Part model, mm, in its own coordinate system. Give positions to 0.01 mm unless a question says otherwise; leave off trailing zeros. Write each loop counter-clockwise with the first axis right and the second up, starting at its lowest first coordinate (ties: lowest second). Pieces come first, ordered by that corner, then holes.
from build123d import *

# Parameters (mm, degrees)
SKETCH1_W           = 25.4
SKETCH1_H           = 25.4
SKETCH1_W_2         = 22.225
SKETCH1_H_2         = 22.225
BOSS_EXTRUDE1_DEPTH = 228.6
SKETCH3_R           = 2.54
CUT_EXTRUDE2_DEPTH  = 232.40501291
SKETCH4_R           = 2.54
CUT_EXTRUDE3_DEPTH  = 232.40501291


with BuildPart() as part:
    # Sketch1 → Boss-Extrude1 (new body)
    with BuildSketch(Plane.XY):
        with Locations((12.7, 12.7)):
            Rectangle(SKETCH1_W, SKETCH1_H)
        with Locations((12.7, 12.7)):
            Rectangle(SKETCH1_W_2, SKETCH1_H_2, mode=Mode.SUBTRACT)
    extrude(amount=BOSS_EXTRUDE1_DEPTH)

    # Sketch3 → Cut-Extrude2 (cut, through all)
    with BuildSketch(Plane(origin=(0, 25.4, 0), x_dir=(1, 0, 0), z_dir=(0, 1, 0))):
        with Locations(Location((12.7, -215.9, 0), (0, 0, 270))):
            Circle(SKETCH3_R)
        with Locations(Location((12.7, -190.5, 0), (0, 0, 270))):
            Circle(SKETCH3_R)
        with Locations(Location((12.7, -12.7, 0), (0, 0, 90))):
            Circle(SKETCH3_R)
        with Locations(Location((12.7, -38.1, 0), (0, 0, 90))):
            Circle(SKETCH3_R)
    extrude(amount=-CUT_EXTRUDE2_DEPTH, mode=Mode.SUBTRACT)

    # Sketch4 → Cut-Extrude3 (cut, through all)
    with BuildSketch(Plane(origin=(25.4, 0, 0), x_dir=(0, 0, -1), z_dir=(1, 0, 0))):
        with Locations((-222.25, 12.7)):
            Circle(SKETCH4_R)
        with Locations((-196.85, 12.7)):
            Circle(SKETCH4_R)
        with Locations(Location((-31.75, 12.7, 0), (0, 0, 180))):
            Circle(SKETCH4_R)
        with Locations(Location((-6.35, 12.7, 0), (0, 0, 180))):
            Circle(SKETCH4_R)
        with Locations((-114.3, 12.7)):
            Circle(SKETCH4_R)
        with Locations((-88.9, 12.7)):
            Circle(SKETCH4_R)
        with Locations((-63.5, 12.7)):
            Circle(SKETCH4_R)
        with Locations((-139.7, 12.7)):
            Circle(SKETCH4_R)
        with Locations((-165.1, 12.7)):
            Circle(SKETCH4_R)
    extrude(amount=-CUT_EXTRUDE3_DEPTH, mode=Mode.SUBTRACT)


solid = part.part
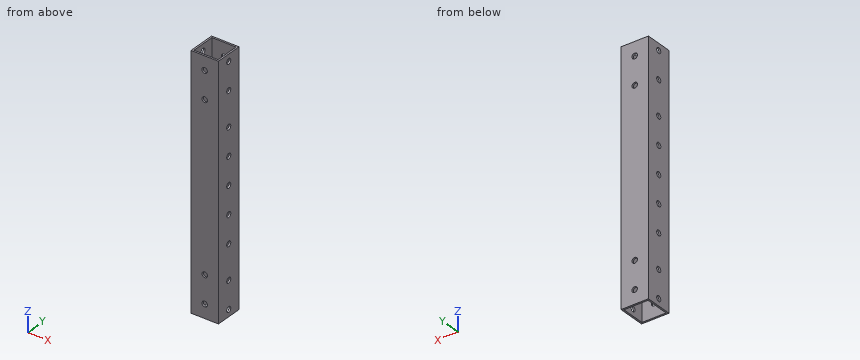
1) Flat gauge pin, fed straight in: P1, Ø10, axis at y = 21.5, z = 160.5, coming from the -X side. Where does the tip first touch, or does it go through?
Check result:
P1: stops at x = 0
2) Saw through at A-A (x = 4). Write the cut outline in (y, z), and give its area (3 significant figures).
Check result:
outline: (0, 0) - (1.59, 0) - (1.59, 228.6) - (0, 228.6) - close; (23.81, 0) - (25.4, 0) - (25.4, 228.6) - (23.81, 228.6) - close
area: 726 mm2
3) Saw through at C-C (z = 38.1). Write the cut outline in (x, y), and give its area (3 significant figures).
Check result:
outline: (0, 0) - (10.16, 0) - (10.16, 1.59) - (1.59, 1.59) - (1.59, 23.81) - (10.16, 23.81) - (10.16, 25.4) - (0, 25.4) - close; (15.24, 0) - (25.4, 0) - (25.4, 25.4) - (15.24, 25.4) - (15.24, 23.81) - (23.81, 23.81) - (23.81, 1.59) - (15.24, 1.59) - close
area: 135 mm2
4) Saw through at D-D (z = 158). Write the cut outline in (x, y), and give its area (3 significant figures).
Check result:
outline: (0, 0) - (25.4, 0) - (25.4, 25.4) - (0, 25.4) - close; hole (1.59, 1.59) - (23.81, 1.59) - (23.81, 23.81) - (1.59, 23.81) - close
area: 151 mm2
5) Drill centre lines: L1, parallel to Y at x = 24.5, z = 88.9; L2, parallel to X at y = 14.5, z = 169. Where is each one in solid material? Low to high.
Check result:
L1: y = 0 to 10.16, 15.24 to 25.4
L2: x = 0 to 1.59, 23.81 to 25.4
